Can you work these out from the model? Positions are in its coordinate system, mm. A direction names the side the tool comes from. Round coordinates to 2 decimals unless told otherwise and drop trailing zeros. Write each loop counter-clockwise with the first axis right and the second up, starting at its lowest first coordinate (ties: lowest second). Pieces come first, ordered by that corner, then holes.
Q1. If we section it at D-D (y = -1.5): Please give me the cut outline in (x, z).
Q2. If we section it at B-B (z = 0.5): Please give me the cut outline in (x, y) (3 decimals).
Q3. I'm going to push flat-ended pins straight in: pin 1 Ø1.8 at (x, z) = (8, 2.5) entering from -Y; pin 2 Ø2 at (x, y) = (15.15, -2.35) entering from -Z; pin 3 Ø3 at (x, y) = (-4.35, -2.35) entering from +Z; pin 4 Ø3 at (x, z) = (8, 2.5) entering from +Y. Where does each tip first touch, or does it pass through?
Q4. We'd pull the mould along X, two halves only. Please class faces 5 (the cylindrical face through (18.4, -2.24, 0.91)), 6 (the cylindrical face through (13.15, -2.3, -0.84)), 7 (the flat face through (-4.6, -4.5, 1.9)), 8 (the cylindrical face through (-2.35, -2.3, 3.13)): +X half, -X half, draft (parallel to the pull), parting line (faces both ways), or undercut.
Q5. Please list where these lines run through material, in increasing order: line 1 along Y through (x, z) = (15.15, 1.4); line 2 along Z through (x, y) = (5.5, -4); line 3 along Y through (x, z) = (1.75, 1).
Q6. If we section it at A-A (x = 15.15): Please give me the cut outline in (y, z).
Q7. For faces 1 (the cylindrical face through (16.997, -3.116, 1.571)), 2 (the cylindrical face through (-2.35, -2.4, -0.84)), 3 (the flat face through (5, 0, 1)), 4 (the flat face through (6, -4.7, 1)), which set-ups out of +Z, -Z, +X, -X, +Y, -Y let a thin tool reach every point of the face, with its end or its side?
Q8. If we section it at C-C (y = 0.5): Please give me the cut outline in (x, z), plus the area to 3 significant figures.
from build123d import *

# Parameters (mm, degrees)
EXTRUDE_4_DEPTH     = 2.5
SKETCH_5_R          = 1.1
EXTRUDE_5_DEPTH     = 2
SKETCH_6_R          = 2
CUT_EXTRUDE_1_DEPTH = 0.666666667
SKETCH_7_R          = 2.35
SKETCH_7_W          = 10.8
SKETCH_7_H          = 4.7
EXTRUDE_6_DEPTH     = 1.5
SKETCH_8_R          = 0.5
EXTRUDE_7_DEPTH     = 1.5


with BuildPart() as part:
    # Эскиз4 → Бобышка-Вытянуть4 (new body)
    with BuildSketch(Plane.XY.offset(1.9)):
        with BuildLine():
            ThreePointArc((0, 0), (-2.35, -2.35), (0, -4.7))
            Line((0, -4.7), (0, 0))
        make_face()
        with BuildLine():
            Line((0, 0), (0, -4.7))
            ThreePointArc((0, -4.7), (1.661700936, -4.011700936), (2.35, -2.35))
            ThreePointArc((2.35, -2.35), (1.661700936, -0.688299064), (0, 0))
        make_face()
        with BuildLine():
            ThreePointArc((2.35, -2.35), (1.661700936, -4.011700936), (0, -4.7))
            Line((0, -4.7), (10.8, -4.7))
            ThreePointArc((10.8, -4.7), (8.45, -2.35), (10.8, 0))
            Line((10.8, 0), (0, 0))
            ThreePointArc((0, 0), (1.661700936, -0.688299064), (2.35, -2.35))
        make_face()
        with BuildLine():
            ThreePointArc((10.8, 0), (8.45, -2.35), (10.8, -4.7))
            Line((10.8, -4.7), (10.8, 0))
        make_face()
        with BuildLine():
            Line((10.8, 0), (10.8, -4.7))
            ThreePointArc((10.8, -4.7), (12.461700936, -4.011700936), (13.15, -2.35))
            ThreePointArc((13.15, -2.35), (12.461700936, -0.688299064), (10.8, 0))
        make_face()
    extrude(amount=EXTRUDE_4_DEPTH)

    # Эскиз5 → Бобышка-Вытянуть5 (add)
    with BuildSketch(Plane(origin=(0, 0, 1.9), x_dir=(-1, 0, 0), z_dir=(0, 0, -1))):
        with BuildLine():
            ThreePointArc((-12.905005568, 0), (-18.4, -2.35), (-12.905005568, -4.7))
            Line((-12.905005568, -4.7), (2.105005568, -4.7))
            ThreePointArc((2.105005568, -4.7), (7.6, -2.35), (2.105005568, 0))
            Line((2.105005568, 0), (-12.905005568, 0))
        make_face()
        with Locations((-15.15, -2.35)):
            Circle(SKETCH_5_R, mode=Mode.SUBTRACT)
        with Locations((4.35, -2.35)):
            Circle(SKETCH_5_R, mode=Mode.SUBTRACT)
    extrude(amount=EXTRUDE_5_DEPTH)

    # Эскиз6 → Вырез-Вытянуть1 (cut)
    with BuildSketch(Plane.XY.offset(1.9)):
        with Locations((15.15, -2.35)):
            Circle(SKETCH_6_R)
        with Locations((-4.35, -2.35)):
            Circle(SKETCH_6_R)
    extrude(amount=-CUT_EXTRUDE_1_DEPTH, mode=Mode.SUBTRACT)

    # Эскиз7 → Бобышка-Вытянуть6 (add)
    with BuildSketch(Plane(origin=(0, 0, -0.1), x_dir=(-1, 0, 0), z_dir=(0, 0, -1))):
        with Locations((-10.8, -2.35)):
            Circle(SKETCH_7_R)
        with Locations((0, -2.35)):
            Circle(SKETCH_7_R)
        with Locations((-5.4, -2.35)):
            Rectangle(SKETCH_7_W, SKETCH_7_H)
    extrude(amount=EXTRUDE_6_DEPTH)

    # Эскиз8 → Бобышка-Вытянуть7 (add)
    with BuildSketch(Plane(origin=(0, 0, -1.6), x_dir=(-1, 0, 0), z_dir=(0, 0, -1))):
        with Locations((-5.4, -2.35)):
            Circle(SKETCH_8_R)
    extrude(amount=EXTRUDE_7_DEPTH)


solid = part.part
A:
1. outline: (-7.49, -0.1) - (-5.05, -0.1) - (-5.05, 1.23) - (-6.16, 1.23) - (-6.16, 1.9) - (-7.49, 1.9) - close; (-3.65, -0.1) - (-2.19, -0.1) - (-2.19, -1.6) - (12.99, -1.6) - (12.99, -0.1) - (14.45, -0.1) - (14.45, 1.23) - (13.34, 1.23) - (13.34, 1.9) - (12.99, 1.9) - (12.99, 4.4) - (-2.19, 4.4) - (-2.19, 1.9) - (-2.54, 1.9) - (-2.54, 1.23) - (-3.65, 1.23) - close; (15.85, -0.1) - (18.29, -0.1) - (18.29, 1.9) - (16.96, 1.9) - (16.96, 1.23) - (15.85, 1.23) - close
2. outline: (-2.105, -4.7) - (12.905, -4.7) arc R3.25 ccw (long way) to (12.905, 0) - (-2.105, 0) arc R3.25 ccw (long way) to start; hole circle Ø2.2 at (-4.35, -2.35); hole circle Ø2.2 at (15.15, -2.35)
3. pin 1: stops at y = -4.7
3. pin 2: passes through
3. pin 3: stops at z = 1.23
3. pin 4: stops at y = 0
4. face 5: undercut
4. face 6: +X half
4. face 7: draft
4. face 8: -X half
5. line 1: y = -5.6 to -4.35, -0.35 to 0.9
5. line 2: z = -1.6 to 4.4
5. line 3: y = -4.7 to 0
6. outline: (-5.6, -0.1) - (-3.45, -0.1) - (-3.45, 1.23) - (-4.35, 1.23) - (-4.35, 1.9) - (-5.6, 1.9) - close; (-1.25, -0.1) - (0.9, -0.1) - (0.9, 1.9) - (-0.35, 1.9) - (-0.35, 1.23) - (-1.25, 1.23) - close
7. face 1: +Z
7. face 2: -Z, -X
7. face 3: +Z, -Z, +Y
7. face 4: +Z, -Z, -Y
8. outline: (-5.91, -0.1) - (-2.79, -0.1) - (-2.79, 1.9) - (-5.91, 1.9) - close; (13.59, -0.1) - (16.71, -0.1) - (16.71, 1.9) - (13.59, 1.9) - close
8. area: 12.5 mm2
